Geometry check sheet. Reference: the model listing, model coordinates, mm. Give positions to 0.01 mm unless a question says otherwise; leave off trailing zeros. Write each loop counter-clockwise with the first axis right and the second up, starting at its lowest first coordinate (ties: lowest second). Pieces come first, ordered by that corner, then holes. Notation, with made-up numbers: (-21.5, 22.25) - (9.5, 22.25) arc R21 ccw to (9.5, 38.25) - close; hole circle Ø6 at (75, -29.75). An arc over 180 degrees is marked (long way). One line per question, with ' | ' between items. Start each with the question number.
Q1. Gauge pin test, flat ends, axial feed: P1, Ø1.5, axis at x = 22, z = 2.5, coming from the +Y side; P2, Ø4, axis at x = 22, y = 43, coming from the -Z side; P3, Ø5, axis at x = 12.7, y = 38.1, coming from the +Z side (3 decimals). Record the tip position at first contact, or that the pin passes through.
Q2. Thickness scan on L1, parallel to X at y = 38.1, z = 1.6; L2, parallel to Y at x = 12.7, z = 1.1; L3, parallel to X at y = 39.5, z = 1.35. Record the ranges inside material, lowest first. Write a range as [from, to].
Q3. Section check C-C on y = 40.5. Record the boundary of the cut face in (x, z) (3 decimals), and give its area (3 significant figures).
Q4. Section check D-D on x = 21.25. Record the boundary of the cut face in (y, z) (3 decimals), and give its area (3 significant figures).
Q5. Section check A-A on z = 2. Record the boundary of the cut face in (x, y).
Q6. Section check B-B on x = 15. Record the boundary of the cut face in (y, z) (3 decimals).
```python
from build123d import *

# Parameters (mm, degrees)
BOSS_EXTRUDE1_DEPTH = 3.175


with BuildPart() as part:
    # Sketch1 → Boss-Extrude1 (new body)
    with BuildSketch(Plane.XY):
        with BuildLine():
            Line((0, 38.1), (0, 0))
            ThreePointArc((0, 0), (3.719743879, 8.980256121), (12.7, 12.7))
            ThreePointArc((12.7, 12.7), (21.680256121, 8.980256121), (25.4, 0))
            Line((25.4, 0), (25.4, 38.1))
            ThreePointArc((25.4, 38.1), (12.7, 50.8), (0, 38.1))
        make_face()
        with BuildLine():
            ThreePointArc((15.9639, 38.1), (15.007925823, 35.792074177), (12.7, 34.8361))
            ThreePointArc((12.7, 34.8361), (10.392074177, 40.407925823), (15.9639, 38.1))
        make_face(mode=Mode.SUBTRACT)
    extrude(amount=BOSS_EXTRUDE1_DEPTH)


solid = part.part
```
Working result:
1) P1: stops at y = 47.49 | P2: stops at z = 0 | P3: passes through
2) L1: x = [0, 9.44], [15.96, 25.4] | L2: y = [12.7, 34.84], [41.36, 50.8] | L3: x = [0.08, 9.75], [15.65, 25.32]
3) outline: (0.229, 0) - (10.488, 0) - (10.488, 3.175) - (0.229, 3.175) - close; (14.912, 0) - (25.171, 0) - (25.171, 3.175) - (14.912, 3.175) - close | area: 65.1 mm2
4) outline: (9.391, 0) - (47.491, 0) - (47.491, 3.175) - (9.391, 3.175) - close | area: 121 mm2
5) outline: (0, 0) arc R12.7 cw to (25.4, 0) - (25.4, 38.1) arc R12.7 ccw to (0, 38.1) - close; hole circle Ø6.53 at (12.7, 38.1)
6) outline: (12.49, 0) - (35.784, 0) - (35.784, 3.175) - (12.49, 3.175) - close; (40.416, 0) - (50.59, 0) - (50.59, 3.175) - (40.416, 3.175) - close
